```python
from build123d import *

# Parameters (mm, degrees)
F0_R     = 42.8625
F0_R_2   = 30.1625
F1_DEPTH = 63.5
F0_R_3   = 63.5
F2_DEPTH = 6.35
F0_R_4   = 2.54
F0_R_5   = 14.2875
F3_DEPTH = 12.7
F5_R     = 2.54
F6_DEPTH = 101.6
F8_R     = 2.54
F9_DEPTH = 101.6


with BuildPart() as f1:
    # F0 (on Front) → F1 (new body)
    with BuildSketch(Plane.XZ):
        Circle(F0_R)
        Circle(F0_R_2, mode=Mode.SUBTRACT)
    extrude(amount=F1_DEPTH)

    # F0 (on Front) → F2 (join)
    with BuildSketch(Plane.XZ):
        Circle(F0_R_3)
        Circle(F0_R, mode=Mode.SUBTRACT)
    extrude(amount=F2_DEPTH)

    # F0 (on Front) → F3 (join)
    with BuildSketch(Plane.XZ):
        Circle(F0_R_2)
        with Locations((-20.62223, -11.90625)):
            Circle(F0_R_4, mode=Mode.SUBTRACT)
        with Locations((0, -23.8125)):
            Circle(F0_R_4, mode=Mode.SUBTRACT)
        with Locations((20.62223, -11.90625)):
            Circle(F0_R_4, mode=Mode.SUBTRACT)
        with Locations((-20.62223, 11.90625)):
            Circle(F0_R_4, mode=Mode.SUBTRACT)
        Circle(F0_R_5, mode=Mode.SUBTRACT)
        with Locations((20.62223, 11.90625)):
            Circle(F0_R_4, mode=Mode.SUBTRACT)
        with Locations((0, 23.8125)):
            Circle(F0_R_4, mode=Mode.SUBTRACT)
    extrude(amount=F3_DEPTH)

    # F5 (on offset) → F6 (cut)
    with BuildSketch(Plane.YZ.offset(45.212)):
        with Locations((-25.4, 0)):
            Circle(F5_R)
        with Locations((-44.45, 0)):
            Circle(F5_R)
    extrude(amount=-F6_DEPTH, mode=Mode.SUBTRACT)

    # F8 (on offset) → F9 (cut)
    with BuildSketch(Plane.XY.offset(44.196)):
        with Locations((0, -25.4)):
            Circle(F8_R)
        with Locations((0, -44.45)):
            Circle(F8_R)
    extrude(amount=-F9_DEPTH, mode=Mode.SUBTRACT)


solid = f1.part
```
Part model, mm, in its own coordinate system. A direction names the side the tool comes from. Give positions to 0.01 mm unless a question says otherwise; leave off trailing zeros. Write each loop counter-clockwise with the first axis right and the second up, starting at its lowest first coordinate (ties: lowest second). Pieces come first, ordered by that corner, then holes. Notation, with made-up numbers: (6.5, -13) -> (28.5, -13) arc R18 cw to (28.5, -7) -> close; hole circle Ø8 at (3.25, -6). An arc over 180 degrees is marked (long way). Put each result on its own line as item: value. Start each with the question number.
Item 1: Cut at A-A (x = 7). List the corners of the cut face in (y, z).
Item 2: Cut at D-D (x = 20). List the corners of the cut face in (y, z), then the cut area to 3 significant figures.
Item 3: Pull direction X, two halves, no side cores. Call faces 3 (the face through (-0.55, -46.93, -36.37)), 4 (the face through (36.549, -27.938, 0.112)), 5 (the face through (23.043, -34.525, 36.142)): pulls with the +X half, pulls with the -X half, needs draft (parallel to the pull), parting line crosses it, or undercut.
Item 4: Cut at C-C (z = -32). List the corners of the cut face in (x, y), then the cut area to 3 significant figures.
Item 5: Cut at B-B (y = -25.4). List the corners of the cut face in (x, z) (1 decimal), then the cut area to 3 significant figures.
Item 6: Pin check, flat tips, straight feed: pin 1 Ø4 at (x, y) = (9.5, -46.5) entering from -Z; pin 2 Ø3 at (x, y) = (36.5, -36.5) entering from -Z; pin 3 Ø6.5 at (x, y) = (0, -25.4) entering from -Z; pin 4 Ø6 at (x, z) = (20.62, -11.91) entering from +Y. Stop position of each tip, or through.
Item 7: Which spindle directions (+Z, -Z, +X, -X, +Y, -Y) get a long thin tool onto all of the face, cutting with end or side? Do faces 1 (the face through (-1, 0, 15)), 2 (the face through (13, -12.7, -6.3)). Say none if no direction does.
Item 8: Wall check: L1, parallel to Z at x = 0, y = -9; L2, parallel to Y at x = 0, z = -35.5; L3, parallel to Y at x = -28.5, z = -55.5. Give the ranges that are in metal, low to high. Write a range as [from, to].
Answer list:
1. outline: (-63.5, -42.29) -> (-6.35, -42.29) -> (-6.35, -63.11) -> (0, -63.11) -> (0, -12.46) -> (-12.7, -12.46) -> (-12.7, -29.34) -> (-63.5, -29.34) -> close; (-63.5, 29.34) -> (-12.7, 29.34) -> (-12.7, 12.46) -> (0, 12.46) -> (0, 63.11) -> (-6.35, 63.11) -> (-6.35, 42.29) -> (-63.5, 42.29) -> close
2. outline: (-63.5, -37.91) -> (-6.35, -37.91) -> (-6.35, -60.27) -> (0, -60.27) -> (0, -14.37) -> (-12.7, -14.37) -> (-12.7, -22.58) -> (-63.5, -22.58) -> close; (-63.5, 22.58) -> (-12.7, 22.58) -> (-12.7, 14.37) -> (0, 14.37) -> (0, 60.27) -> (-6.35, 60.27) -> (-6.35, 37.91) -> (-63.5, 37.91) -> close; (-12.7, -9.44) -> (0, -9.44) -> (0, 9.44) -> (-12.7, 9.44) -> close
2. area: 2,680 mm2
3. face 3: undercut
3. face 4: needs draft
3. face 5: parting line crosses it
4. outline: (-54.85, -6.35) -> (-28.52, -6.35) -> (-28.52, -63.5) -> (28.52, -63.5) -> (28.52, -6.35) -> (54.85, -6.35) -> (54.85, 0) -> (-54.85, 0) -> close; hole circle Ø5.08 at (0, -44.45); hole circle Ø5.08 at (0, -25.4)
4. area: 3,920 mm2
5. outline: (-42.8, -2.5) arc R42.9 ccw to (-2.5, -42.8) -> (-2.5, -30.1) arc R30.2 cw to (-30.1, -2.5) -> close; (-42.8, 2.5) -> (-30.1, 2.5) arc R30.2 cw to (-2.5, 30.1) -> (-2.5, 42.8) arc R42.9 ccw to start; (2.5, -42.8) arc R42.9 ccw to (42.8, -2.5) -> (30.1, -2.5) arc R30.2 cw to (2.5, -30.1) -> close; (2.5, 30.1) arc R30.2 cw to (30.1, 2.5) -> (42.8, 2.5) arc R42.9 ccw to (2.5, 42.8) -> close
5. area: 2,660 mm2
6. pin 1: stops at z = -42.2
6. pin 2: stops at z = -24.74
6. pin 3: stops at z = -42.86
6. pin 4: stops at y = 0
7. face 1: +Z, -Z, +X, -X, +Y
7. face 2: -Y
8. L1: z = [-42.86, -26.35], [-21.27, -14.29], [14.29, 21.27], [26.35, 42.86]
8. L2: y = [-63.5, -46.99], [-41.91, -27.94], [-22.86, 0]
8. L3: y = [-6.35, 0]
